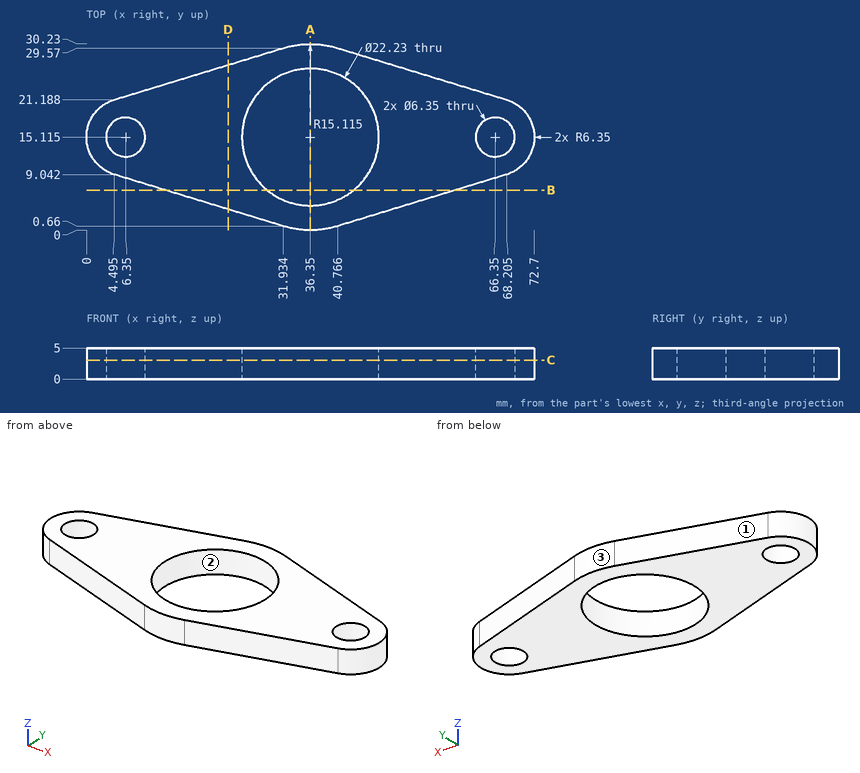
Geometry check sheet. Reference: drawing and pictorial views, mm from the part's lowest x, y, z. Coordinates: 2 decimals unless noted, no trailing zeros. Order: outer loops, then holes, each group sorted by start corner. A loop starts at its lowest first (then second) coordinate and runs counter-clockwise, first axis right, second up. Notation, with made-up numbers: (-12, 0.25) -> (-4, 0.25) arc R20 cw to (-4, 15.25) -> close; hole circle Ø7 at (59.5, 24). An arc over 180 degrees is marked (long way). Write item = value, one per line. Start each with the question number.
1) Mould release check, pull along X, two halves, no side actions. Record for the marked faces 1, 2 and 3: +X half, -X half, draft (parallel to the pull), parting line (faces both ways), or undercut.
2) Go/stop test with flat-tipped pins: P1, Ø1.5, axis at x = 62, z = 0.5, coming from the -Y side; P2, Ø3, axis at x = 42.5, z = 1, coming from the +Y side. Record where each tip stops, or that it passes through.
3) Cross-section at C-C (z = 3.05). State how many separate pieces and enclosed holes the cut face has, then the cut area to 3 significant figures.
4) Cross-section at A-A (x = 36.35). Enter the section's corners in (y, z), then the cut area to 3 significant figures.
5) Cross-section at D-D (x = 23). Enter the section's corners in (y, z).
6) Material ranges on L1, parallel to X at y = 15, z = 1.45 (1 decimal); L2, parallel to Y at x = 36.35, z = 1.25; L3, parallel to X at y = 18, z = 2.4 (1 decimal), recorded low to high.
7) Cross-section at B-B (y = 6.5). Enter the section's corners in (x, z) (1 decimal).
Ans:
q1.face_1 = -X half
q1.face_2 = undercut
q1.face_3 = parting line
q2.P1 = 6.92
q2.P2 = 29.5
q3.separate_pieces = 1
q3.enclosed_holes = 3
q3.area = 1,020 mm²
q4.outline = (0, 0) -> (4, 0) -> (4, 5) -> (0, 5) -> close; (26.23, 0) -> (30.23, 0) -> (30.23, 5) -> (26.23, 5) -> close
q4.area = 40.0 mm²
q5.outline = (3.39, 0) -> (26.84, 0) -> (26.84, 5) -> (3.39, 5) -> close
q6.L1 = 0 to 3.2, 9.5 to 25.2, 47.5 to 63.2, 69.5 to 72.7
q6.L2 = 0 to 4, 26.23 to 30.23
q6.L3 = 0.7 to 5, 7.7 to 25.6, 47.1 to 65, 67.7 to 72
q7.outline = (12.8, 0) -> (29.3, 0) -> (29.3, 5) -> (12.8, 5) -> close; (43.4, 0) -> (59.9, 0) -> (59.9, 5) -> (43.4, 5) -> close
